from build123d import *

# Parameters (mm, degrees)
SKETCH1_W               = 292.1
SKETCH1_H               = 57.15
BOSS_EXTRUDE1_DEPTH     = 6.35
SKETCH3_W               = 31.75
SKETCH3_H               = 25.4
CUT_EXTRUDE2_DEPTH      = 1
CUT_EXTRUDE2_DEPTH_BACK = 7.35


with BuildPart() as part:
    # Sketch1 → Boss-Extrude1 (new body)
    with BuildSketch(Plane.XY):
        with Locations((146.05, 28.575)):
            Rectangle(SKETCH1_W, SKETCH1_H)
    extrude(amount=BOSS_EXTRUDE1_DEPTH)

    # Sketch3 → Cut-Extrude2 (cut, two sides)
    with BuildSketch(Plane.XY.offset(6.35)) as cut_extrude2_sk:
        with Locations((15.875, 44.45)):
            Rectangle(SKETCH3_W, SKETCH3_H)
    extrude(amount=CUT_EXTRUDE2_DEPTH, mode=Mode.SUBTRACT)
    extrude(cut_extrude2_sk.sketch, amount=-CUT_EXTRUDE2_DEPTH_BACK, mode=Mode.SUBTRACT)


solid = part.part
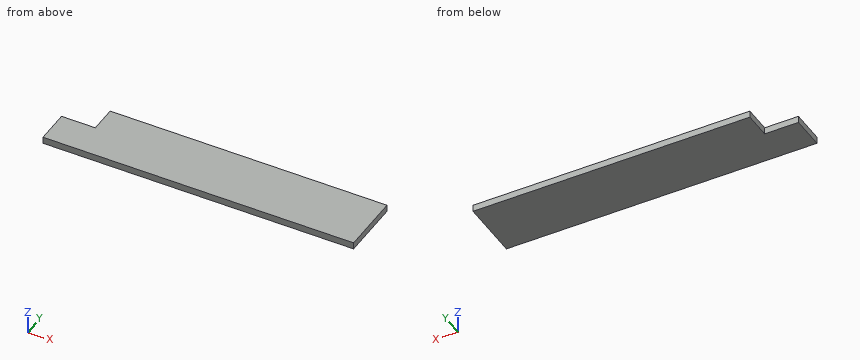
Can you work these out from the model? Positions are in its coordinate system, mm. Round coordinates to 2 decimals unless told otherwise and drop trailing zeros. Order: outer loops, then holes, each group sorted by start corner. A loop starts at its lowest first (then second) coordinate and runs counter-clockwise, first axis right, second up. Notation, with made-up numbers: M -2,9.5 L 36,9.5 A15 ccw 36,32.5 Z; hole C 1.25,16 d1. An arc over 180 degrees is marked long. Use a Markdown table: item, result.
1) Imagine slicing it at A-A (z = 5.25). List the corners of the cut face in (x, y) for me, then the cut area to 3 significant figures.
Geometry says:
| item | result |
|---|---|
| outline | M 0,0 L 292.1,0 L 292.1,57.15 L 31.75,57.15 L 31.75,31.75 L 0,31.75 Z |
| area | 15,900 mm² |
2) I'm going to push flat-ended pins straight in: P1, Ø3, axis at y = 43.5, z = 4, coming from the -X side; P2, Ø1.9, axis at x = 8.5, z = 2, coming from the +Y side. Where does each tip first touch, or does it pass through?
Geometry says:
| item | result |
|---|---|
| P1 | stops at x = 31.75 |
| P2 | stops at y = 31.75 |
3) If I drill on line 1 along X through (y, z) = (38.5, 4.5); line 2 along Y through (x, z) = (30.5, 4.5), over which ranges is the centre line in solid material (lowest first)?
Geometry says:
| item | result |
|---|---|
| line 1 | x = 31.75 to 292.1 |
| line 2 | y = 0 to 31.75 |
